Read the model definition and answer for the solid it produces. Units are mm, in the model's axes. Face numbers are marked on the shaded views. A direction names the side the tool comes from. Give positions to 0.01 mm unless a question says otherwise; leave off trailing zeros. Loops run counter-clockwise (first coordinate to the right, second up) from the corner with the lowest first, then second, coordinate; pieces in that order, holes last. Notation, with made-up numbers: (-18, 54.5) -> (18, 54.5) arc R16 ccw to (18, 66.5) -> close; hole circle Ø2 at (25.25, -27). An arc over 180 degrees is marked (long way). Return JSON: item names as keys, results as strings. Group by question number.
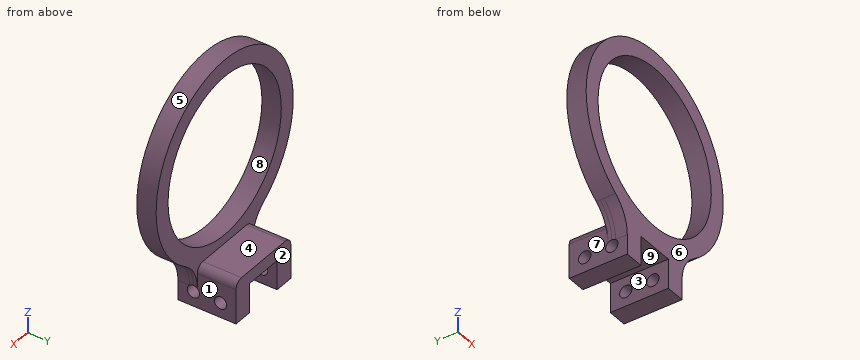
from build123d import *

# Parameters (mm, degrees)
SKETCH_1_R          = 25
SKETCH_1_R_2        = 20.65
EXTRUDE_1_DEPTH     = 5
EXTRUDE_2_DEPTH     = 15
SKETCH_3_R          = 1.6
CUT_EXTRUDE_1_DEPTH = 35.982946782
FILLET_1_R          = 10
FILLET_2_R          = 2


with BuildPart() as part:
    # 草图1 → 凸台-拉伸1 (new body)
    with BuildSketch(Plane(origin=(0, 0, 0), x_dir=(1, 0, 0), z_dir=(0, 1, 0))):
        Circle(SKETCH_1_R)
        Circle(SKETCH_1_R_2, mode=Mode.SUBTRACT)
    extrude(amount=EXTRUDE_1_DEPTH)

    # 草图2 → 凸台-拉伸2 (add)
    with BuildSketch(Plane(origin=(0, 0, 0), x_dir=(1, 0, 0), z_dir=(0, 1, 0))):
        Polygon((-5, 33.807000777), (-9.982946782, 33.807000777), (-9.982946782, 22.896387671), (9.982946782, 22.896387671), (9.982946782, 33.807000777), (5, 33.807000777), (5, 26.192999223), (-5, 26.192999223), align=None)
    extrude(amount=EXTRUDE_2_DEPTH)

    # 草图3 → 切除-拉伸1 (cut, through all)
    with BuildSketch(Plane.ZY.offset(9.982946782)):
        with Locations((-30, 4)):
            Circle(SKETCH_3_R)
        with Locations((-30, 11)):
            Circle(SKETCH_3_R)
    extrude(amount=-CUT_EXTRUDE_1_DEPTH, mode=Mode.SUBTRACT)

    # 圆角1
    fillet_1_edges = [part.edges().sort_by_distance(p)[0] for p in [
        (9.982946782, 2.5, -22.920313557),
        (-9.982946782, 2.5, -22.920313557),
    ]]
    fillet(fillet_1_edges, radius=FILLET_1_R)

    # 圆角2
    fillet_2_edges = [part.edges().sort_by_distance(p)[0] for p in [
        (-9.982946782, 10, -22.896387671),
        (9.982946782, 10, -22.896387671),
    ]]
    fillet(fillet_2_edges, radius=FILLET_2_R)


solid = part.part
1. Determine the mould class of the marked faces 6, 7, 8 and 9 for opening direction X: pulls with the +X half, pulls with the -X half, needs draft (parallel to the pull), parting line crosses it, or undercut.
2. Straight lines are drawn through the part: line 1 (Y direction, x = 7.95, z = -30); line 2 (X direction, y = 1.1, z = 0); line 3 (Z direction, x = -14.5, y = 0.5). For each, find the intervals that lie inside material, in ascending order. Write a range as from..to.
3. Flat-ended cylindrical pins translate along their axes: pin 1 Ø5 at (y, z) = (4, -30) entering from -X; pin 2 Ø3 at (x, y) = (-2.5, 6) entering from -Z; pin 3 Ø25 at (x, z) = (0, 0) entering from +Y; pin 4 Ø3.5 at (y, z) = (11, -30) entering from +X. Find the tip coordinate at first contact, or state that the pin passes through.
4. Which of the six approach directions +Z, -Z, +X, -X, +Y, -Y give full straight-line access (tool end or side, diameter ignored) to the marked faces 1, 2, 3, 4 and 5?
5. Section B-B on z = 0 is taken. Determine the outline of the cut face in (x, y), then the cut area to 3 significant figures.
6. Section D-D on z = -30 is taken. Determine the outline of the cut face in (x, y), then the cut area to 3 significant figures.
7. Section A-A on x = -6.5 is taken. Determine the outline of the cut face in (y, z).
8. Section C-C on y = 8 is taken. Determine the outline of the cut face in (x, z), then the cut area to 3 significant figures.
Completed:
{
 "1": {"face 6": "needs draft", "face 7": "pulls with the -X half", "face 8": "undercut", "face 9": "undercut"},
 "2": {"line 1": "y = 0..2.4, 5.6..9.4, 12.6..15", "line 2": "x = -25..-20.65, 20.65..25", "line 3": "z = -20.37..-14.7, 14.7..20.37"},
 "3": {"pin 1": "stops at x = -10.05", "pin 2": "stops at z = -26.19", "pin 3": "passes through", "pin 4": "stops at x = 9.98"},
 "4": {"face 1": "-Z, +X, +Y", "face 2": "+Z, -Z, +X, -X, +Y", "face 3": "-Z, +Y, -Y", "face 4": "+Z, +X, -X, +Y", "face 5": "+Y, -Y"},
 "5": {"outline": "(-25, 0) -> (-20.65, 0) -> (-20.65, 5) -> (-25, 5) -> close; (20.65, 0) -> (25, 0) -> (25, 5) -> (20.65, 5) -> close", "area": "43.5 mm²"},
 "6": {"outline": "(-9.98, 0) -> (-5, 0) -> (-5, 2.4) -> (-9.98, 2.4) -> close; (-9.98, 5.6) -> (-5, 5.6) -> (-5, 9.4) -> (-9.98, 9.4) -> close; (-9.98, 12.6) -> (-5, 12.6) -> (-5, 15) -> (-9.98, 15) -> close; (5, 0) -> (9.98, 0) -> (9.98, 2.4) -> (5, 2.4) -> close; (5, 5.6) -> (9.98, 5.6) -> (9.98, 9.4) -> (5, 9.4) -> close; (5, 12.6) -> (9.98, 12.6) -> (9.98, 15) -> (5, 15) -> close", "area": "85.7 mm²"},
 "7": {"outline": "(0, -33.81) -> (15, -33.81) -> (15, -22.9) -> (5, -22.9) -> (5, -19.6) -> (0, -19.6) -> close; (0, 19.6) -> (5, 19.6) -> (5, 24.14) -> (0, 24.14) -> close; hole circle Ø3.2 at (4, -30); hole circle Ø3.2 at (11, -30)"},
 "8": {"outline": "(-9.98, -33.81) -> (-5, -33.81) -> (-5, -26.19) -> (5, -26.19) -> (5, -33.81) -> (9.98, -33.81) -> (9.98, -24.9) arc R2 ccw to (7.98, -22.9) -> (-7.98, -22.9) arc R2 ccw to (-9.98, -24.9) -> close", "area": "140 mm²"}
}
